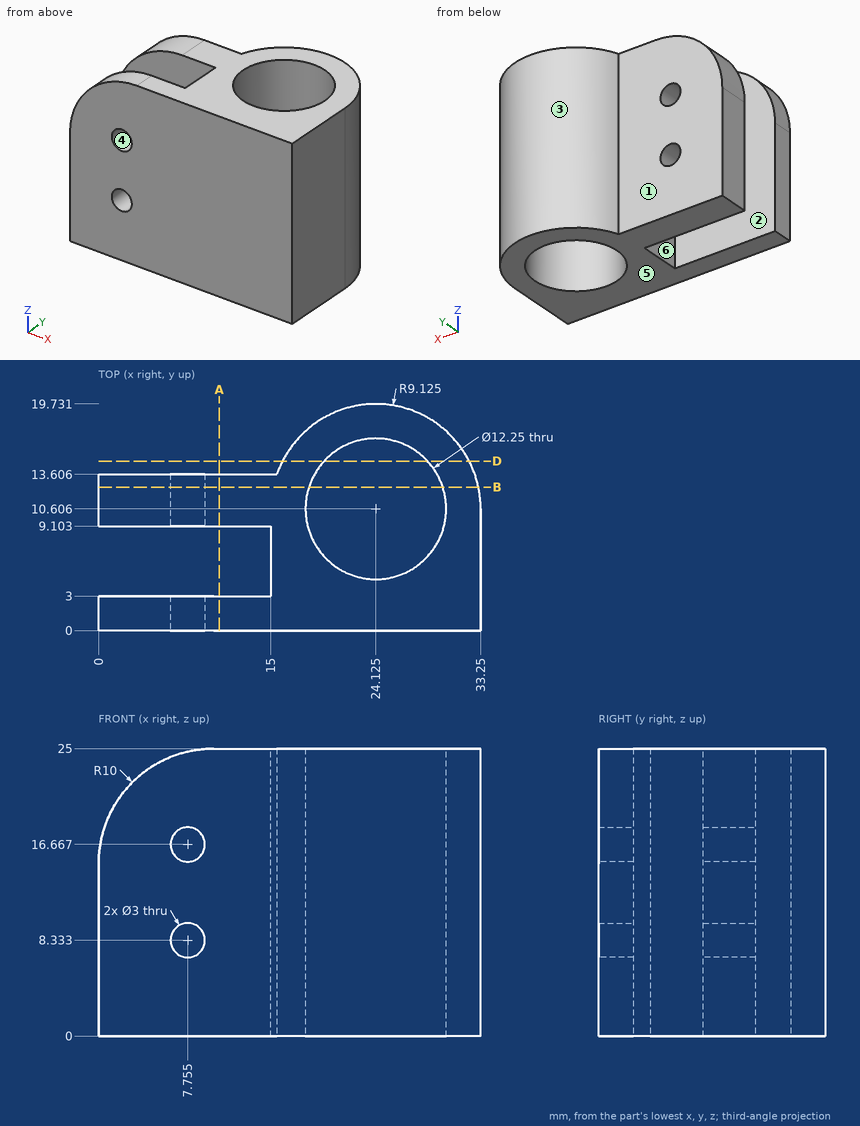
Check sheet for the drawn part. Datum: minimum x, y, z corner. Units: mm. A direction names the side the tool comes from. Give positions to 0.01 mm unless a question says otherwise; leave off trailing zeros. Order: outer loops, then holes, each group sorted by start corner. A loop starts at its lowest first (then second) coordinate and runs counter-clockwise, first axis right, second up. Notation, with made-up numbers: (89.25, 33) -> (134.25, 33) arc R8 ccw to (134.25, 41) -> close; hole circle Ø8 at (22.25, 67). An arc over 180 degrees is marked (long way). Answer as CSV lines item,"result".
Q1. Depth check by flat-ended pin: pin 1 (6 mm diameter, centred on x = 22.5, y = 10.5, fed in from -Z); pin 2 (4.5 mm diameter, centred on x = 10.5, z = 8.5, fed in from +Y); pin 3 (4 mm diameter, centred on x = 20.5, z = 15, fed in from +Y) (1 decimal). Enter the tip coordinate at first touch or a pass-through.
Solutions:
pin 1,"passes through"
pin 2,"stops at y = 13.61"
pin 3,"stops at y = 19.6"
Q2. Sectioned sample at A-A on x = 10.5. Record the cut outline in (y, z), plus the area to 3 significant figures.
Solutions:
outline,"(0, 0) -> (3, 0) -> (3, 25) -> (0, 25) -> close; (9.1, 0) -> (13.61, 0) -> (13.61, 25) -> (9.1, 25) -> close"
area,"188 mm²"
Q3. Sectioned sample at B-B on y = 12.5. Count the separate pieces of the cut face and the enclosed holes in it.
Solutions:
separate pieces,"2"
enclosed holes,"2"
Q4. Release check for a two-part mould opening along Z. For the marked faces 4, 5 and 6 record: +Z half, -Z half, draft (parallel to the pull), parting line (faces both ways), or undercut.
Solutions:
face 4,"undercut"
face 5,"-Z half"
face 6,"draft"
Q5. Scan lines: probe 1 along Y at (x, z) = (9, 4); probe 2 along X at (y, z) = (11.25, 15.75) (1 decimal); probe 3 along X at (y, z) = (3.5, 3.5). Record each from-to range of solid material in increasing order.
Solutions:
probe 1,"y = 0 to 3, 9.1 to 13.61"
probe 2,"x = 0 to 6.6, 8.9 to 18, 30.2 to 33.2"
probe 3,"x = 15 to 33.25"
Q6. Sectioned sample at D-D on y = 14.75. Record the cut outline in (x, z) (1 decimal), plus the area to 3 significant figures.
Solutions:
outline,"(16, 0) -> (19.6, 0) -> (19.6, 25) -> (16, 25) -> close; (28.6, 0) -> (32.3, 0) -> (32.3, 25) -> (28.6, 25) -> close"
area,"181 mm²"
Q7. Access from +Z, -Z, +X, -X, +Y, -Y to the whole of each face (thin tool, end or side, straight path). Record for the marked faces 1, 2 and 3.
Solutions:
face 1,"+Z, -Z, -X, +Y"
face 2,"+Z, -Z, -X"
face 3,"+Z, -Z, +Y"
